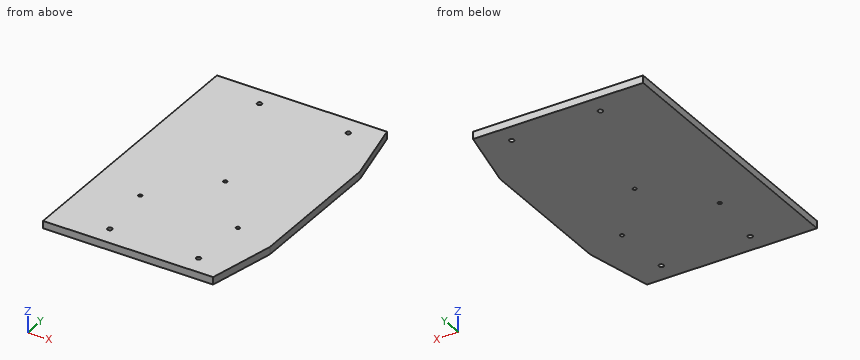
Autodesk Fusion 360 part; units mm, degrees
sketch "Sketch1" plane through (0, 0, 0) normal (0, 0, 1) x (1, 0, 0)
  line L0 (125, 90) -> (-125, 90)
  line L1 (-125, 90) -> (-125, -90)
  line L2 (-125, -90) -> (125, -90)
  line L3 (125, -90) -> (125, 90)
  line L4 (125, 90) -> (-125, -90) construction
  line L5 (-125, 90) -> (125, -90) construction
  line L6 (0, 90) -> (-97, 90)
  line L7 (0, 0) -> (0, 90)
  line L8 (0, 90) -> (97, 90)
  line L9 (-97, 90) -> (-97, 77)
  circle A0 centre (-97, 77) radius 1.6
  line L10 (0, 90) -> (-37, 90)
  line L11 (-37, 90) -> (-37, 77)
  circle A1 centre (-37, 77) radius 1.6
  line L12 (97, 90) -> (97, 77)
  line L13 (0, 90) -> (-115, 90)
  line L14 (-115, 90) -> (-125, 44.9959)
  line L15 (-125, 44.9959) -> (-125, 90)
  line L16 (-125, 90) -> (-115, 90)
  line L17 (0, 0) -> (0, -90)
  line L18 (115, 90) -> (125, 44.9959)
  line L19 (125, 44.9959) -> (125, 90)
  line L20 (125, 90) -> (115, 90)
  line L21 (-125, -44.9959) -> (-125, -90)
  line L22 (-125, -90) -> (-115, -90)
  line L23 (125, -44.9959) -> (125, -90)
  line L24 (125, -90) -> (115, -90)
  line L25 (-97, 77) -> (-97, -84)
  line L26 (-97, -84) -> (-97, -90)
  line L27 (-97, -84) -> (-97, -97)
  line L28 (-97, -97) -> (-125.0061, -97)
  line L29 (-125.0061, -97) -> (-125, -90)
  line L30 (-97, -97) -> (125, -97)
  line L31 (125, -97) -> (125, -90)
  line L32 (-37, 77) -> (-37, -84)
  circle A2 centre (-97, -84) radius 1.6
  circle A3 centre (-37, -84) radius 1.6
  circle A4 centre (97, -84) radius 1.6
  circle A5 centre (37, -84) radius 1.6
  circle A6 centre (97, 77) radius 1.6
  circle A7 centre (37, 77) radius 1.6
  line L33 (0, -97) -> (0, 90)
  line L34 (-125.0061, -97) -> (-125.0061, -3.5)
  line L35 (-125.0061, -3.5) -> (125, -3.5)
  line L36 (115, 90) -> (125, 44.9959)
  line L37 (-115, -97) -> (-125, -51.9959)
  line L38 (115, -97) -> (125, -51.9959)
  dimension "d1" = 250
  dimension "d2" = 180
  dimension "d3" = 97
  dimension "d4" = 13
  dimension "d5" = 3.2
  dimension "d6" = 37
  dimension "d7" = 13
  dimension "d8" = 3.2
  dimension "d9" = 115
  dimension "d14" = 161
  dimension "d15" = 13
  dimension "d16" = 161
  dimension "d17" = 3.2
  dimension "d18" = 3.2
  dimension "d19" = 93.5
extrude "Extrude3" add sketch "Sketch1" against normal blind 5 contours A6 | L0 L3 L7 L8 L17 L18 L33 L35 L36 | L2 L3 L17 L23 L24 L33 L35 L38 | L2 L24 L30 L33 L38 | A4 | A5 | A7
extrude "Extrude4" cut sketch "Sketch1" against normal blind 10 contours A6 | L11 A1 L32 | L9 A0 L25 | L25 L26 L27 A2 | A4 | A5 | A7 picked at (-36.3624, 76.1483) picked at (-96.2477, 77.7523) picked at (-96.2477, -84.7523)
sketch "Sketch3" plane through (0, 0, 0) normal (0, 0, 1) x (-1, 0, 0)
  circle A0 centre (-97, 84) radius 1.6
  circle A1 centre (-97, -77) radius 1.6
  circle A2 centre (-37, 84) radius 1.6
  circle A3 centre (-37, -77) radius 1.6
  line L0 (0, 97) -> (-115, 97)
  line L1 (-115, 97) -> (-125, 51.9959)
  line L2 (-125, 51.9959) -> (-125, -44.9959)
  line L3 (-125, -44.9959) -> (-115, -90)
  line L4 (-115, -90) -> (0, -90)
  line L5 (0, -90) -> (0, 97)
  line L6 (0, 97) -> (-115, 97)
  line L7 (-32.4552, 44.0647) -> (-98.4552, 44.0647)
  circle A4 centre (-32.4552, 44.0647) radius 1.25
  circle A5 centre (-98.4552, 44.0647) radius 1.25
  line L8 (-65.4552, 44.0647) -> (-65.4552, 5.0647)
  circle A6 centre (-65.4552, 5.0647) radius 1.25
  dimension "d28" = 115
  dimension "d29" = 60
  dimension "d30" = 66
  dimension "d31" = 2.5
  dimension "d32" = 2.5
  dimension "d33" = 39
  dimension "d34" = 2.5
extrude "Extrude6" cut sketch "Sketch3" against normal blind 30 contours A5 | A4 | A6
Read the model definition and answer for the solid it produces. Units are mm, in the model's axes. Round coordinates to 2 decimals unless told otherwise and drop trailing zeros. Loops run counter-clockwise (first coordinate to the right, second up) from the corner with the lowest first, then second, coordinate; pieces in that order, holes last.
Q1. Consider probe 1 along Y at (x, z) = (37, -1.85); probe 2 along Y at (x, z) = (97.5, -3.35); probe 3 along X at (y, z) = (77, -1.85). Determine where each line is inside the solid, lowest interval first.
Q2. Section A-A on z = -4.1 is taken. Write down the section's boundary in (x, y), and give its area (3 significant figures).
Q3. Section B-B on y = -66.5 is taken. Write down the section's boundary in (x, z), and give its area (3 significant figures).
Output:
1. probe 1: y = -97 to -85.6, -82.4 to 75.4, 78.6 to 90
1. probe 2: y = -97 to -85.52, -82.48 to -44.87, -43.26 to 75.48, 78.52 to 90
1. probe 3: x = 0 to 35.4, 38.6 to 95.4, 98.6 to 117.89
2. outline: (0, -97) - (115, -97) - (125, -52) - (125, 45) - (115, 90) - (0, 90) - close; hole circle Ø2.5 at (32.46, -44.06); hole circle Ø3.2 at (37, -84); hole circle Ø3.2 at (37, 77); hole circle Ø2.5 at (65.46, -5.06); hole circle Ø3.2 at (97, -84); hole circle Ø3.2 at (97, 77); hole circle Ø2.5 at (98.46, -44.06)
2. area: 22,900 mm2
3. outline: (0, -5) - (121.78, -5) - (121.78, 0) - (0, 0) - close
3. area: 609 mm2
